Autodesk Inventor part; units mm, degrees
ref_plane "Combination_Module_XY" through (0, 0, 0) normal (1, 0, 0) x (0, 0, -1)
ref_plane "Combination_Module_YZ" through (0, 0, 0) normal (0, 0, -1) x (0, 1, 0)
ref_plane "Combination_Module_ZX" through (0, 0, 0) normal (0, 1, 0) x (1, 0, 0)
sketch "Sketch_1" plane through (0, 0, 0) normal (0, 0, 1) x (1, 0, 0)
  line L0 (24, 0) -> (0, 0)
  line L1 (0, 4) -> (24, 4)
  line L2 (24, 4) -> (24, 6.6)
  arc A0 (24, 6.6) -> (23.1, 7.5) centre (23.1, 6.6) ccw
  line L3 (23.1, 7.5) -> (6.6, 7.5)
  line L4 (6.6, 7.5) -> (6.6, 7.25)
  line L5 (6.6, 7.25) -> (5, 7.25)
  line L6 (5, 7.25) -> (5, 15.5)
  line L7 (5, 15.5) -> (4.5, 16)
  line L8 (4.5, 16) -> (0.5, 16)
  line L9 (0.5, 16) -> (0, 15.5)
  line L10 (0, 15.5) -> (0, 4)
revolve "Revolution1" add sketch "Sketch_1" angle 360 about axis through (24, 0, 0) along (1, 0, 0)
sketch "Sketch_3" plane through (0, 0, 0) normal (1, 0, 0) x (0, 1, 0)
  line L0 (-32, 32) -> (-32, -32)
  line L1 (-32, -32) -> (32, -32)
  line L2 (32, -32) -> (32, 32)
  line L3 (32, 32) -> (-32, 32)
  line L4 (12.0727, 10.5) -> (-12.0727, 10.5)
  arc A0 (-12.0727, 10.5) -> (-12.0727, -10.5) centre (0, 0) ccw
  line L5 (-12.0727, -10.5) -> (12.0727, -10.5)
  arc A1 (12.0727, -10.5) -> (12.0727, 10.5) centre (0, 0) ccw
extrude "Extrusion1" cut sketch "Sketch_3" along normal blind 5
sketch "Sketch3" plane through (0, -11.4018, -10.5) normal (-1, 0, 0) x (0, 0, 1)
  point P0 (10.5, 23.4018)
hole "Hole1" at (0, 12, 0) direction (1, 0, 0) diameter 3.5 depth 5 counterbore diameter 6 counterbore depth 3.1
sketch "Sketch4" plane through (0, -11.4018, -10.5) normal (-1, 0, 0) x (0, 0, 1)
  point P0 (10.5, -0.5982)
hole "Hole2" at (0, -12, 0) direction (1, 0, 0) diameter 3.5 depth 5 counterbore diameter 6 counterbore depth 3.1
ref_plane "Combination_Module_XY" through (0, 0, 0) normal (1, 0, 0) x (0, 0, -1)
ref_plane "Combination_Module_YZ" through (0, 0, 0) normal (0, 0, -1) x (0, 1, 0)
ref_plane "Combination_Module_ZX" through (0, 0, 0) normal (0, 1, 0) x (1, 0, 0)
properties part number "C-LHFC8"
Input: part model. Units: mm. Frame: model coordinates. A direction names the side the tool comes from. Give positions to 0.01 mm unless a question says otherwise; leave off trailing zeros. Loops run counter-clockwise (first coordinate to the right, second up) from the corner with the lowest first, then second, coordinate; pieces in that order, holes last.
1) Section query C-C on z = 0. Count the separate pieces of the cut face and the enclosed holes in it, and give its area (3 significant figures).
A:
separate pieces: 4
enclosed holes: 0
area: 201 mm2
2) Reachability of faces 4 (the cylindrical face through (12.168, -0.867, -3.905)), 5 (the cylindrical face through (1.57, 14.93, -0.65)) from +Z, -Z, +X, -X, +Y, -Y: full face, straight path, thin tool, end or side. Return the list, or none.
A:
face 4: +X, -X
face 5: -X
3) Line query: L1, parallel to Z at x = 17, y = 0; L2, parallel to Z at x = 3.75, y = 1; L3, parallel to X at y = -5.5, z = -7. Output: solid intervals per line, ascending.
A:
L1: z = -7.5 to -4, 4 to 7.5
L2: z = -10.5 to -3.87, 3.87 to 10.5
L3: x = 0 to 5
4) Section query A-A on x = 3.5. Return the cut outline in (y, z), and give its area (3 significant figures).
A:
outline: (-12.07, -10.5) - (12.07, -10.5) arc R16 ccw to (12.07, 10.5) - (-12.07, 10.5) arc R16 ccw to start; hole circle Ø3.5 at (-12, 0); hole circle Ø8 at (0, 0); hole circle Ø3.5 at (12, 0)
area: 551 mm2
5) Section query B-B on y = 0. Return the cut outline in (x, z).
A:
outline: (0, -10.5) - (5, -10.5) - (5, -7.25) - (6.6, -7.25) - (6.6, -7.5) - (23.1, -7.5) arc R0.9 ccw to (24, -6.6) - (24, -4) - (0, -4) - close; (0, 4) - (24, 4) - (24, 6.6) arc R0.9 ccw to (23.1, 7.5) - (6.6, 7.5) - (6.6, 7.25) - (5, 7.25) - (5, 10.5) - (0, 10.5) - close
6) Section query D-D on x = 15.75. Return the cut outline in (y, z).
A:
outline: circle Ø15 at (0, 0); hole circle Ø8 at (0, 0)
7) Mould query, pull axis X, two halves, no side actions, for faces 1 (the cylindrical face through (14.734, -7.493, -0.33)), 2 (the flat face through (3.1, 14, 0)), 3 (the cylindrical face through (5.79, 3.35, 6.43)). Classes: released by +X, released by -X, zero draft, split by the parting line, or undercut.
A:
face 1: zero draft
face 2: released by -X
face 3: undercut
8) Contact query for flat-ended pins moving along their axis: pin 1 (5 mm diameter, centred on y = -2.5, z = 0.5, fed in from -X); pin 2 (1.8 mm diameter, centred on y = -11.5, z = -1, fed in from -X); pin 3 (1 mm diameter, centred on x = 10, z = 5.5, fed in from -Y); pin 4 (7 mm diameter, centred on y = 12, z = 0, fed in from +X). Output: stop coordinate, or through.
A:
pin 1: stops at x = 0
pin 2: stops at x = 3.1
pin 3: stops at y = -5.59
pin 4: stops at x = 5
